from build123d import *

# Parameters (mm, degrees)
F0_R      = 1.8
F1_DEPTH  = 2
F2_R      = 4.99999
F3_W      = 70
F3_H      = 5
F4_DEPTH  = 10
F5_W      = 70
F5_H      = 3
F6_DEPTH  = 6
F8_W      = 9
F8_H      = 2
F9_DEPTH  = 8
F10_W     = 9
F10_H     = 2
F11_DEPTH = 10
F7_R      = 1.5
F12_DEPTH = 12.001
F13_R     = 1


# Not quite as in the source:
# - a fillet or chamfer is up to 0.001 mm smaller than in the source, because OpenCascade refuses the exact size


with BuildPart() as f1:
    # F0 (on Top) → F1 (new body)
    with BuildSketch(Plane.XY):
        Polygon((-22.5, 10), (-35, 10), (-35, -10), (35, -10), (35, 10), (22.5, 10), (22.5, 0), (0, 0), (-22.5, 0), align=None)
        with Locations((-28.5, 4)):
            Circle(F0_R, mode=Mode.SUBTRACT)
        with Locations((28.5, 4)):
            Circle(F0_R, mode=Mode.SUBTRACT)
    extrude(amount=F1_DEPTH)

    # F2 (radius 5 in the source; OpenCascade refuses exactly that, so slightly less here)
    f2_edges = [f1.edges().sort_by_distance(p)[0] for p in [
        (22.5, 10, 1),
        (35, 10, 1),
        (-22.5, 10, 1),
        (-35, 10, 1),
        (-22.5, 0, 1),
        (22.5, 0, 1),
    ]]
    fillet(f2_edges, radius=F2_R)

    # F3 (on face) → F4 (join)
    with BuildSketch(Plane.XY.offset(2)):
        with Locations((0, -7.5)):
            Rectangle(F3_W, F3_H)
    extrude(amount=F4_DEPTH)

    # F5 (on face) → F6 (join)
    with BuildSketch(Plane.XZ.offset(10)):
        with Locations((0, 1.5)):
            Rectangle(F5_W, F5_H)
    extrude(amount=F6_DEPTH)

    # F8 (on face) → F9 (join)
    with BuildSketch(Plane.XZ.offset(10)):
        with Locations((13.5, 11)):
            Rectangle(F8_W, F8_H)
    extrude(amount=F9_DEPTH)

    # F10 (on face) → F11 (join)
    with BuildSketch(Plane(origin=(0, 0, 10), x_dir=(1, 0, 0), z_dir=(0, 0, -1))):
        with Locations((13.5, 17)):
            Rectangle(F10_W, F10_H)
    extrude(amount=F11_DEPTH)

    # F7 (on face) → F12 (cut, through all)
    with BuildSketch(Plane(origin=(0, 0, 0), x_dir=(1, 0, 0), z_dir=(0, 0, -1))):
        with Locations((13.5, 12.5)):
            Circle(F7_R)
    extrude(amount=-F12_DEPTH, mode=Mode.SUBTRACT)

    # F13
    f13_edges = [f1.edges().sort_by_distance(p)[0] for p in [
        (9, -18, 6),
        (18, -18, 6),
    ]]
    fillet(f13_edges, radius=F13_R)


solid = f1.part
Design review of the part built by this model. Coordinates are the model's own, in mm. A direction names the side the tool comes from. Round coordinates to 2 decimals unless told otherwise and drop trailing zeros. Write each loop counter-clockwise with the first axis right and the second up, starting at its lowest first coordinate (ties: lowest second). Pieces come first, ordered by that corner, then holes. Notation, with made-up numbers: (0, -10) -> (42, -10) arc R21 cw to (42, 7) -> close; hole circle Ø5 at (76, -32). An arc over 180 degrees is marked (long way). One line per question, with ' | ' between items.
(1) Machinability: for faces 1 (the flat face through (0, -5, 7)), 2 (the cylindrical face through (21, 1.43, 1.01)), 3 (the flat face through (12, -14, 10)), 4 (the flat face through (18, -16.3, 9.1)), 5 (the flat face through (-13, -16, 2)), which of the approach directions +Z, -Z, +X, -X, +Y, -Y give a long, thin tool a straight path to every point of the face, cutting with its end or side? Answer none if there is none.
Result sheet:
face 1: +Z, +X, -X, +Y | face 2: +Z, -Z, +Y | face 3: +X, -X | face 4: +Z, +X, -Y | face 5: +Z, -Z, -X, -Y
(2) Take a section at B-B, the plane x = 28.5. State the section outline as (y, z) points, and give its area (3 significant figures).
Result sheet:
outline: (-16, 0) -> (2.2, 0) -> (2.2, 2) -> (-5, 2) -> (-5, 12) -> (-10, 12) -> (-10, 3) -> (-16, 3) -> close; (5.8, 0) -> (10, 0) -> (10, 2) -> (5.8, 2) -> close | area: 101 mm2
(3) Take a section at C-C, the plane x = 16. State the section outline as (y, z) points.
Result sheet:
outline: (-18, 0) -> (0, 0) -> (0, 2) -> (-5, 2) -> (-5, 12) -> (-18, 12) -> close; hole (-16, 3) -> (-10, 3) -> (-10, 10) -> (-16, 10) -> close
(4) Wall thickness on line 1 (Y direction, x = 13.5, z = 10.85); line 2 (X direction, y = -12.5, z = 10.6); line 3 (X direction, y = -12.5, z = 1.8): over which ranges is each line inside the solid? List them lowest first. Write a range as [from, to].
Result sheet:
line 1: [-18, -14], [-11, -5] | line 2: [9, 12], [15, 18] | line 3: [-35, 12], [15, 35]
(5) Take a section at A-A, the plane y = 1. State the section outline as (x, z) points.
Result sheet:
outline: (-35, 0) -> (-20.5, 0) -> (-20.5, 2) -> (-35, 2) -> close; (20.5, 0) -> (35, 0) -> (35, 2) -> (20.5, 2) -> close
(6) Insertion check: P1, Ø4.5, axis at x = -0.5, z = 5.5, coming from the -Y side; P2, Ø4, axis at x = -20.5, z = 6, coming from the +Y side; P3, Ø2.5, axis at x = 23.5, z = 1.5, coming from the -Y side. Each pin has a flat end and moves straight along its axis. Give the tip position at first contact, or say it passes through.
Result sheet:
P1: y = -10 | P2: y = -5 | P3: y = -16
(7) Draft analysis for pull direction X (two halves, no side actions). For faces 6 (the flat face through (0, -4, 0)), 7 (the flat face through (35, -5.4, 3.2)), 8 (the cylindrical face through (12, -12.57, 10.99)), state which applies: released by +X, released by -X, zero draft, split by the parting line, or undercut.
Result sheet:
face 6: zero draft | face 7: released by +X | face 8: undercut
(8) Take a section at D-D, the plane z = 5.75. State the section outline as (x, y) points.
Result sheet:
outline: (-35, -10) -> (35, -10) -> (35, -5) -> (-35, -5) -> close; (9, -17) arc R1 ccw to (10, -18) -> (17, -18) arc R1 ccw to (18, -17) -> (18, -16) -> (9, -16) -> close
